Solid Edge part; units mm, degrees
sketch "Sketch1" plane through (0, 0, 0) normal (0, 0, 1) x (1, 0, 0)
  line L0 (-35, -35) -> (35, -35)
  line L1 (35, -35) -> (35, 35)
  line L2 (35, 35) -> (-35, 35)
  line L3 (-35, 35) -> (-35, -35)
  dimension "D1" = 35
  dimension "D2" = 35
extrude "Protrusion1" add sketch "Sketch1" along normal blind 5
sketch "Sketch2" plane through (0, 0, 5) normal (0, 0, 1) x (1, 0, 0)
  circle A0 centre (25, -32.5) radius 1.875
  circle A1 centre (-25, -32.5) radius 1.875
  circle A2 centre (-25, 32.5) radius 1.875
  circle A3 centre (25, 32.5) radius 1.875
  dimension "D1" = 25
  dimension "D2" = 25
extrude "Cutout1" cut sketch "Sketch2" against normal through all
chamfer "Fase_1" distance 0.5 angle 45 3 edges at (-26.875, -32.5, 5) (-26.875, 32.5, 5) (23.125, 32.5, 5)
sketch "Sketch3" plane through (35, 0, 2.5) normal (1, 0, 0) x (0, 1, 0)
  line L0 (-53, 12.5) -> (-75, 12.5)
  line L1 (-75, 12.5) -> (-75, 17.5)
  line L2 (-75, 17.5) -> (75, 17.5)
  line L3 (75, 17.5) -> (75, 12.5)
  line L4 (75, 12.5) -> (53, 12.5)
  line L5 (43, 2.5) -> (53, 12.5)
  line L6 (43, -2.5) -> (43, 2.5)
  line L7 (35, -2.5) -> (43, -2.5)
  line L8 (35, -2.5) -> (35, 2.5)
  line L9 (35, 2.5) -> (45, 12.5)
  line L10 (45, 12.5) -> (4, 12.5)
  line L11 (4, 12.5) -> (4, 2.5)
  line L12 (4, -2.5) -> (4, 2.5)
  line L13 (-4, -2.5) -> (4, -2.5)
  line L14 (-4, 2.5) -> (-4, -2.5)
  line L15 (-4, 2.5) -> (-4, 12.5)
  line L16 (-4, 12.5) -> (-45, 12.5)
  line L17 (-45, 12.5) -> (-35, 2.5)
  line L18 (-35, 2.5) -> (-35, -2.5)
  line L19 (-35, -2.5) -> (-43, -2.5)
  line L20 (-43, -2.5) -> (-43, 2.5)
  line L21 (-43, 2.5) -> (-53, 12.5)
  dimension "D1" = 75
  dimension "D2" = 75
  dimension "D3" = 4
  dimension "D4" = 35
extrude "Extrusionsausprägung_2" add sketch "Sketch3" against normal blind 100
sketch "Sketch4" plane through (-15, -75, 32.5) normal (0, -1, 0) x (-1, 0, 0)
  line L0 (-50, 32.5) -> (-50, 27.5)
  line L1 (-50, 27.5) -> (-40, 17.5)
  line L2 (-40, 17.5) -> (-40, 12.5)
  dimension "D1" = 50
extrude "Cutout2" cut sketch "Sketch4" against normal through all material side at (35.05, -75, 2.5)
sketch "Sketch5" plane through (-27.5, -75, 32.5) normal (0, -1, 0) x (1, 0, 0)
  line L0 (-7.5, -32.5) -> (-7.5, -27.5)
  line L1 (-7.5, -27.5) -> (-17.5, -17.5)
  line L2 (-17.5, -17.5) -> (-17.5, -12.5)
extrude "Cutout3" cut sketch "Sketch5" against normal through all material side at (-35.05, -75, 2.5)
sketch "Sketch6" plane through (-10, 0, 20) normal (0, 0, 1) x (1, 0, 0)
  circle A0 centre (22.5, 62.5) radius 2.5
  circle A1 centre (-22.5, 62.5) radius 2.5
  circle A2 centre (-22.5, -62.5) radius 2.5
  circle A3 centre (22.5, -62.5) radius 2.5
  circle A4 centre (22.5, 0) radius 2.5
  dimension "D1" = 22.5
  dimension "D2" = 22.5
extrude "Cutout4" cut sketch "Sketch6" against normal through all
chamfer "Fase_2" distance 0.5 angle 45 5 edges at (-35, -62.5, 20) (10, -62.5, 20) (10, 0, 20) (-35, 62.5, 20) (10, 62.5, 20)
sketch "Sketch7" plane through (-10, 0, 20) normal (0, 0, 1) x (0, 1, 0)
  line L0 (-44, 35) -> (-9, 35)
  line L1 (-9, 35) -> (-9, 10)
  line L2 (-9, 10) -> (-44, 10)
  line L3 (-44, 10) -> (-44, 35)
  line L4 (9, 35) -> (44, 35)
  line L5 (44, 35) -> (44, 10)
  line L6 (44, 10) -> (9, 10)
  line L7 (9, 10) -> (9, 35)
  dimension "D1" = 44
  dimension "D2" = 44
extrude "Cutout5" cut sketch "Sketch7" against normal up to vertex (5 mm away)
sketch "Sketch8" plane through (-10, 0, 20) normal (0, 0, 1) x (0, 1, 0)
  line L0 (-9, 25) -> (9, 25)
  line L1 (9, 25) -> (9, 35)
  line L2 (9, 35) -> (-9, 35)
  line L3 (-9, 35) -> (-9, 25)
extrude "Cutout6" cut sketch "Sketch8" against normal through all
sketch "Sketch9" plane through (0, 0, 0) normal (0, 0, -1) x (0, 1, 0)
  circle A0 centre (0, 12.5) radius 10
extrude "Cutout7" cut sketch "Sketch9" against normal up to vertex (15 mm away)
properties material "Nylon, allgemein"
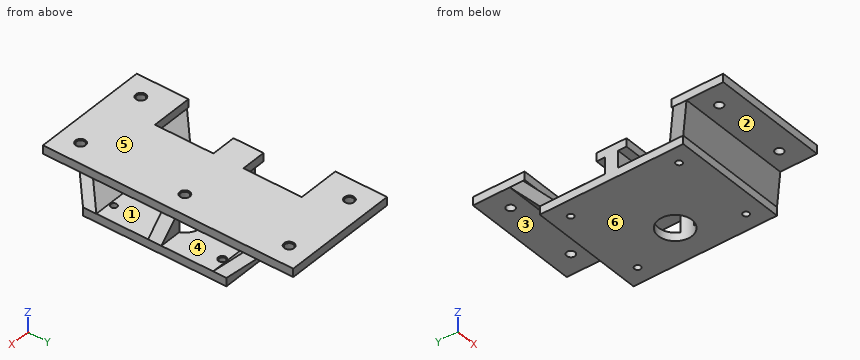
The listing builds one solid part. Answer for the finished solid, in the listing's coordinates (mm). Face numbers are marked on the shaded views. A direction names the side the tool comes from. Round coordinates to 2 decimals unless told otherwise and drop trailing zeros. Order: outer loops, then holes, each group sorted by start corner. A loop starts at its lowest first (then second) coordinate and runs counter-clockwise, first axis right, second up. Notation, with made-up numbers: M 56.5,-7.5 L 104.5,-7.5 A31 ccw 104.5,16.5 Z; hole C 16,-9.75 d9. An arc over 180 degrees is marked long. Answer in a Markdown table with one row per item. Add a question column.
1) The part is cut by section B-B on z = 12.5. Determine the outline of the cut face in (x, y), plus the area to 3 significant figures.
2) The part is cut by section C-C on y = -62.5. Determine the outline of the cut face in (x, z).
3) The part is cut by section D-D on x = -32.5. Count the separate pieces of the cut face and the enclosed holes in it, plus the area to 3 significant figures.
4) Flat-ended cylindrical pins translate along their axes: pin 1 Ø2.5 at (y, z) = (27.5, 17) entering from -X; pin 2 Ø3 at (x, z) = (26, 10.5) entering from +Y; pin 3 Ø24 at (x, y) = (-25.5, 67.5) entering from -Z. Find the tip coordinate at first contact, or state that the pin passes through.
5) Consider line 1 along Y through (x, z) = (12.5, 18.65); line 2 along Y through (x, z) = (-32.5, 17.7); line 3 along Y through (x, z) = (25, 1) (3 decimals). Determine where each line is inside the solid, lowest interval first. Write a range as from..to.
6) Determine the mould class of the marked faces 4, 5 and 6 for opening direction Z: pulls with the +Z half, pulls with the -Z half, needs draft (parallel to the pull), parting line crosses it, or undercut.
7) Which of the six approach directions +Z, -Z, +X, -X, +Y, -Y give full straight-line access (tool end or side, diameter ignored) to the marked faces 1, 2 and 3?
8) The part is cut by section A-A on y = -32.5. Determine the outline of the cut face in (x, z) (3 decimals), plus the area to 3 significant figures.
Findings below:
| question | item | result |
|---|---|---|
| 1 | outline | M -42.5,-50.5 L 27.5,-50.5 L 27.5,-42.5 L -42.5,-42.5 Z; M -42.5,42.5 L 27.5,42.5 L 27.5,50.5 L -42.5,50.5 Z; M -35,-4 L 3.33,-4 A10 cw 3.33,4 L -35,4 Z; M 21.67,-4 L 27.5,-4 L 27.5,4 L 21.67,4 A10 cw Z |
| 1 | area | 1,460 mm² |
| 2 | outline | M -45,15 L -35,15 L -35,19.5 L -35.5,20 L -45,20 Z; M -30,15 L 10,15 L 10,19.5 L 9.5,20 L -29.5,20 L -30,19.5 Z; M 15,15 L 25,15 L 25,20 L 15.5,20 L 15,19.5 Z |
| 3 | separate pieces | 3 |
| 3 | enclosed holes | 0 |
| 3 | area | 1,020 mm² |
| 4 | pin 1 | stops at x = -20 |
| 4 | pin 2 | stops at y = 50 |
| 4 | pin 3 | stops at z = 15 |
| 5 | line 1 | y = -75..-65, -60..-2.5, 2.5..60, 65..75 |
| 5 | line 2 | y = -75..-65, -60..-44, -9..9, 44..60, 65..75 |
| 5 | line 3 | y = -43..-34.375, -30.625..30.625, 34.375..43 |
| 6 | face 4 | undercut |
| 6 | face 5 | pulls with the +Z half |
| 6 | face 6 | pulls with the -Z half |
| 7 | face 1 | +X, -X |
| 7 | face 2 | -Z, +X, -X, -Y |
| 7 | face 3 | -Z, +X, -X, +Y |
| 8 | outline | M -35,0 L -26.875,0 L -26.875,4.5 L -27.375,5 L -35,5 Z; M -23.125,0 L 23.125,0 L 23.125,5 L -22.625,5 L -23.125,4.5 Z; M -20,15 L 25,15 L 25,20 L -20,20 Z; M 26.875,0 L 35,0 L 35,5 L 26.875,5 Z |
| 8 | area | 537 mm² |
